The listing builds one solid part. Answer for the finished solid, in the listing's coordinates (mm). A direction names the side the tool comes from. Coordinates: 2 decimals unless noted, no trailing zeros. Write each loop counter-clockwise with the first axis right and the second up, starting at its lowest first coordinate (ties: lowest second). Pieces come first, ordered by that corner, then holes.
(1) Given P1, Ø12.5, axis at x = 165, y = 47, coming from the -Z side; P2, Ø6, axis at x = 85, y = 46, coming from the -Z side; P3, Ø10, axis at x = 50, y = 17.5, coming from the +Z side; P4, Ø5.5, axis at x = 155.5, y = 45, coming from the +Z side, each flat-ended and moving along its own axis, determine where each tip first touches the part or whether it passes through.
(2) For a pull along X with two mould halves and no side action, classify faces 1 (the cylindrical face through (-152.16, 46.05, -4.93)), 2 (the flat face through (-171, 47, -5)), 3 (the flat face through (-159, 57, -10)) as +X half, -X half, draft (parallel to the pull), parting line (faces both ways), or undercut.
(3) The part is cut by section B-B on y = 45. Determine the outline of the cut face in (x, z), plus the area to 3 significant figures.
(4) The part is cut by section C-C on x = -155.5. Determine the outline of the cut face in (y, z), plus the area to 3 significant figures.
(5) The part is cut by section A-A on z = -6.5. Determine the outline of the cut face in (x, y).
(6) Straight lines are drawn through the part: line 1 (Z direction, x = 154.5, y = 54.5); line 2 (Y direction, x = 155.5, z = -4.25); line 3 (Z direction, x = -9, y = 88). For each, find the intervals that lie inside material, in ascending order.
(7) Which of the six approach directions +Z, -Z, +X, -X, +Y, -Y give full straight-line access (tool end or side, diameter ignored) to faces 4 (the flat face through (-2, 0, -15)), 5 (the flat face through (159, 57, -10)), 6 (the cylindrical face through (143.008, 56.695, -0.163))?
(8) The part is cut by section D-D on y = 79.5. Determine the outline of the cut face in (x, z).
from build123d import *

# Parameters (mm, degrees)
EXTRUDE_1_DEPTH     = 115
SKETCH_4_R          = 3.5
CUT_EXTRUDE_2_DEPTH = 208.464142308
FILLET_1_R          = 20


with BuildPart() as part:
    # Эскиз1 → Вытянуть-Тонкостенный1 (new body)
    with BuildSketch(Plane(origin=(0, 0, 0), x_dir=(1, 0, 0), z_dir=(0, 1, 0))):
        with BuildLine():
            Line((-171, 0), (-146.383337508, 0))
            ThreePointArc((-146.383337508, 0), (-143.05426157, 0.158684678), (-139.755372679, 0.633299806))
            ThreePointArc((-139.755372679, 0.633299806), (0, 13.986878572), (139.755372679, 0.633299806))
            ThreePointArc((139.755372679, 0.633299806), (143.05426157, 0.158684678), (146.383337508, 0))
            Line((146.383337508, 0), (171, 0))
            Line((171, 0), (171, 10))
            Line((171, 10), (146.383337508, 10))
            ThreePointArc((146.383337508, 10), (144.005426124, 10.113346198), (141.649076916, 10.452357004))
            ThreePointArc((141.649076916, 10.452357004), (0, 23.986878572), (-141.649076916, 10.452357004))
            ThreePointArc((-141.649076916, 10.452357004), (-144.005426124, 10.113346198), (-146.383337508, 10))
            Line((-146.383337508, 10), (-171, 10))
            Line((-171, 10), (-171, 0))
        make_face()
    extrude(amount=EXTRUDE_1_DEPTH)

    # Эскиз4 → Вырез-Вытянуть2 (cut, through all)
    with BuildSketch(Plane.XY):
        with Locations((-155.5, 45)):
            Circle(SKETCH_4_R)
        with Locations((155.5, 45)):
            Circle(SKETCH_4_R)
    extrude(amount=-CUT_EXTRUDE_2_DEPTH, mode=Mode.SUBTRACT)

    # Скругление1
    fillet_1_edges = [part.edges().sort_by_distance(p)[0] for p in [
        (171, 115, -5),
        (-171, 115, -5),
    ]]
    fillet(fillet_1_edges, radius=FILLET_1_R)


solid = part.part
Model answer:
1. P1: stops at z = -10
1. P2: stops at z = -19.48
1. P3: stops at z = -11.93
1. P4: passes through
2. face 1: undercut
2. face 2: -X half
2. face 3: draft
3. outline: (-171, -10) - (-159, -10) - (-159, 0) - (-171, 0) - close; (-152, -10) - (-146.38, -10) arc R25 cw to (-141.65, -10.45) arc R748 ccw to (141.65, -10.45) arc R25 cw to (146.38, -10) - (152, -10) - (152, 0) - (146.38, 0) arc R35 ccw to (139.76, -0.63) arc R738 cw to (-139.76, -0.63) arc R35 ccw to (-146.38, 0) - (-152, 0) - close; (159, -10) - (171, -10) - (171, 0) - (159, 0) - close
3. area: 3,300 mm2
4. outline: (0, -10) - (41.5, -10) - (41.5, 0) - (0, 0) - close; (48.5, -10) - (114.49, -10) - (114.49, 0) - (48.5, 0) - close
4. area: 1,070 mm2
5. outline: (-171, 0) - (-104.86, 0) - (-104.86, 115) - (-151, 115) arc R20 ccw to (-171, 95) - close; (104.86, 0) - (171, 0) - (171, 95) arc R20 ccw to (151, 115) - (104.86, 115) - close; hole circle Ø7 at (-155.5, 45); hole circle Ø7 at (155.5, 45)
6. line 1: z = -10 to 0
6. line 2: y = 0 to 41.5, 48.5 to 114.49
6. line 3: z = -23.93 to -13.93
7. face 4: +Z, -Z, +X, -X, -Y
7. face 5: -Z, +X, +Y, -Y
7. face 6: +Z, +Y, -Y
8. outline: (-171, -10) - (-146.38, -10) arc R25 cw to (-141.65, -10.45) arc R748 ccw to (141.65, -10.45) arc R25 cw to (146.38, -10) - (171, -10) - (171, 0) - (146.38, 0) arc R35 ccw to (139.76, -0.63) arc R738 cw to (-139.76, -0.63) arc R35 ccw to (-146.38, 0) - (-171, 0) - close
